Geometry check sheet. Reference: the model listing, model coordinates, mm. A direction names the side the tool comes from. Round coordinates to 2 decimals unless told otherwise and drop trailing zeros. Write each loop counter-clockwise with the first axis right and the second up, starting at its lowest first coordinate (ties: lowest second). Pieces come first, ordered by that corner, then holes. Notation, with made-up numbers: (-9.75, -14) - (42.25, -14) arc R4 cw to (42.25, -8) - close; hole circle Ø7 at (-14.5, 30). An arc over 180 degrees is marked (long way). Return JSON: item names as keys, results as strings.
```python
from build123d import *

# Parameters (mm, degrees)
SKETCH1_W           = 75
SKETCH1_H           = 180
BOSS_EXTRUDE1_DEPTH = 6
FILLET1_R           = 10
SKETCH2_R           = 10.5
SKETCH2_R_2         = 1.25
SKETCH2_R_3         = 1.65
CUT_EXTRUDE1_DEPTH  = 10
CUT_EXTRUDE2_DEPTH  = 3
SKETCH5_R           = 3.5
SKETCH5_W           = 47
SKETCH5_H           = 60
CUT_EXTRUDE3_DEPTH  = 3
FILLET2_R           = 10
CHAMFER1_SIZE       = 3
SKETCH6_W           = 5
SKETCH6_H           = 10
BOSS_EXTRUDE2_DEPTH = 6
CHAMFER2_SIZE       = 6


with BuildPart() as part:
    # Sketch1 → Boss-Extrude1 (new body)
    with BuildSketch(Plane(origin=(0, 0, 0), x_dir=(1, 0, 0), z_dir=(0, 1, 0))):
        Rectangle(SKETCH1_W, SKETCH1_H)
    extrude(amount=BOSS_EXTRUDE1_DEPTH)

    # Fillet1
    fillet1_edges = [part.edges().sort_by_distance(p)[0] for p in [
        (-37.5, 3, -90),
        (37.5, 3, -90),
        (37.5, 3, 90),
        (-37.5, 3, 90),
    ]]
    fillet(fillet1_edges, radius=FILLET1_R)

    # Sketch2 → Cut-Extrude1 (cut)
    with BuildSketch(Plane(origin=(0, 6, 0), x_dir=(1, 0, 0), z_dir=(0, 1, 0))):
        with Locations(Location((0, 0, 0), (0, 0, 270))):
            Circle(SKETCH2_R)
        with Locations(Location((-11, 8, 0), (0, 0, 270))):
            Circle(SKETCH2_R_2)
        with Locations(Location((11, 8, 0), (0, 0, 270))):
            Circle(SKETCH2_R_2)
        with Locations(Location((-11, -32, 0), (0, 0, 270))):
            Circle(SKETCH2_R_2)
        with Locations(Location((11, -32, 0), (0, 0, 270))):
            Circle(SKETCH2_R_2)
        with Locations(Location((-28, -70, 0), (0, 0, 270))):
            Circle(SKETCH2_R_3)
        with Locations(Location((28, -70, 0), (0, 0, 270))):
            Circle(SKETCH2_R_3)
        with Locations(Location((-28, 70, 0), (0, 0, 270))):
            Circle(SKETCH2_R_3)
        with Locations(Location((28, 70, 0), (0, 0, 270))):
            Circle(SKETCH2_R_3)
        with Locations(Location((-28, 10, 0), (0, 0, 270))):
            Circle(SKETCH2_R_3)
        with Locations(Location((-28, -10, 0), (0, 0, 270))):
            Circle(SKETCH2_R_3)
        with Locations(Location((28, 10, 0), (0, 0, 270))):
            Circle(SKETCH2_R_3)
        with Locations(Location((28, -10, 0), (0, 0, 270))):
            Circle(SKETCH2_R_3)
        with Locations(Location((-28, 30, 0), (0, 0, 270))):
            Circle(SKETCH2_R_3)
        with Locations(Location((28, 30, 0), (0, 0, 270))):
            Circle(SKETCH2_R_3)
        with Locations(Location((28, -30, 0), (0, 0, 270))):
            Circle(SKETCH2_R_3)
        with Locations(Location((-28, -30, 0), (0, 0, 270))):
            Circle(SKETCH2_R_3)
    extrude(amount=-CUT_EXTRUDE1_DEPTH, mode=Mode.SUBTRACT)

    # Sketch4 → Cut-Extrude2 (cut)
    with BuildSketch(Plane.XZ):
        Polygon((-28, 6.766838493), (-25.2, 8.383419246), (-25.2, 11.616580754), (-28, 13.233161507), (-30.8, 11.616580754), (-30.8, 8.383419246), align=None)
        Polygon((-27.920583163, -13.232185994), (-25.161136401, -11.547315999), (-25.240553238, -8.315130005), (-28.079416837, -6.767814006), (-30.838863599, -8.452684001), (-30.759446762, -11.684869995), align=None)
        Polygon((28, -13.233161507), (30.8, -11.616580754), (30.8, -8.383419246), (28, -6.766838493), (25.2, -8.383419246), (25.2, -11.616580754), align=None)
        Polygon((28, 6.766838493), (30.8, 8.383419246), (30.8, 11.616580754), (28, 13.233161507), (25.2, 11.616580754), (25.2, 8.383419246), align=None)
        Polygon((28, 66.766838493), (30.8, 68.383419246), (30.8, 71.616580754), (28, 73.233161507), (25.2, 71.616580754), (25.2, 68.383419246), align=None)
        Polygon((-28, 66.766838493), (-25.2, 68.383419246), (-25.2, 71.616580754), (-28, 73.233161507), (-30.8, 71.616580754), (-30.8, 68.383419246), align=None)
        Polygon((28, -73.233161507), (30.8, -71.616580754), (30.8, -68.383419246), (28, -66.766838493), (25.2, -68.383419246), (25.2, -71.616580754), align=None)
        Polygon((-28, -73.233161507), (-25.2, -71.616580754), (-25.2, -68.383419246), (-28, -66.766838493), (-30.8, -68.383419246), (-30.8, -71.616580754), align=None)
    extrude(amount=-CUT_EXTRUDE2_DEPTH, mode=Mode.SUBTRACT)

    # Sketch5 → Cut-Extrude3 (cut)
    with BuildSketch(Plane(origin=(0, 6, 0), x_dir=(1, 0, 0), z_dir=(0, 1, 0))):
        with Locations((-11, 8)):
            Circle(SKETCH5_R)
        with Locations((11, 8)):
            Circle(SKETCH5_R)
        with Locations((0, 50)):
            Rectangle(SKETCH5_W, SKETCH5_H)
        with Locations((0, -50)):
            Rectangle(SKETCH5_W, SKETCH5_H)
    extrude(amount=-CUT_EXTRUDE3_DEPTH, mode=Mode.SUBTRACT)

    # Fillet2
    fillet2_edges = [part.edges().sort_by_distance(p)[0] for p in [
        (-7.57722899, 4.5, -7.268810139),
        (-9.249798037, 4.5, -4.969027699),
        (9.249798037, 4.5, -4.969027699),
        (7.57722899, 4.5, -7.268810139),
    ]]
    fillet(fillet2_edges, radius=FILLET2_R)

    # Chamfer1
    chamfer1_edges = [part.edges().sort_by_distance(p)[0] for p in [
        (0, 3, 80),
        (0, 3, -80),
        (0, 3, -20),
        (0, 3, 20),
    ]]
    chamfer(chamfer1_edges, length=CHAMFER1_SIZE - 0.0001)  # a hair under: the kernel refuses the full size

    # Sketch6 → Boss-Extrude2 (add)
    with BuildSketch(Plane(origin=(0, 6, 0), x_dir=(1, 0, 0), z_dir=(0, 1, 0))):
        with Locations((-21, 85)):
            Rectangle(SKETCH6_W, SKETCH6_H)
        with Locations((21, -85)):
            Rectangle(SKETCH6_W, SKETCH6_H)
        with Locations((21, 85)):
            Rectangle(SKETCH6_W, SKETCH6_H)
        with Locations((-21, -85)):
            Rectangle(SKETCH6_W, SKETCH6_H)
    extrude(amount=BOSS_EXTRUDE2_DEPTH)

    # Chamfer2
    chamfer2_edges = [part.edges().sort_by_distance(p)[0] for p in [
        (21, 12, 90),
        (-21, 12, -90),
        (21, 12, -90),
        (-21, 12, 90),
    ]]
    chamfer(chamfer2_edges, length=CHAMFER2_SIZE)


solid = part.part
```
(1) Section check C-C, the plane z = 70. Enter the section's corners in (x, y), plus the area to 3 significant figures.
Response values:
{"outline": "(-37.5, 0) - (-30.8, 0) - (-30.8, 3) - (-29.65, 3) - (-29.65, 6) - (-37.5, 6) - close; (-26.35, 3) - (-25.2, 3) - (-25.2, 0) - (25.2, 0) - (25.2, 3) - (26.35, 3) - (26.35, 6) - (23.5, 6) - (23.5, 3) - (-23.5, 3) - (-23.5, 6) - (-26.35, 6) - close; (29.65, 3) - (30.8, 3) - (30.8, 0) - (37.5, 0) - (37.5, 6) - (29.65, 6) - close", "area": "256 mm^2"}
(2) Release check for a two-part mould opening along X. For faces 5 (the face through (-25.2, 1, -70)), 6 (the face through (21, 9, 87)), 7 (the face through (37.5, 3, 1)), 8 (the face through (29.636, 3.042, -30.215)) record: pulls with the +X half, pulls with the -X half, needs draft (parallel to the pull), parting line crosses it, or undercut.
Response values:
{"face 5": "undercut", "face 6": "needs draft", "face 7": "pulls with the +X half", "face 8": "undercut"}
(3) Material ranges on line 1 along X through (y, z) = (1.2, 30); line 2 along Z through (x, y) = (-7, 5.25); line 3 along Z through (x, y) = (7, 5.5), recorded low to high. Write a range as [from, to].
Response values:
{"line 1": "x = [-37.5, -29.65], [-26.35, 26.35], [29.65, 37.5]", "line 2": "z = [-90, -79.25], [-20.75, -10.21], [7.83, 20.75], [79.25, 90]", "line 3": "z = [-90, -79.5], [-20.5, -10.21], [7.83, 20.5], [79.5, 90]"}
(4) Gauge pin test, flat ends, axial feed: pin 1 (14 mm diameter, centred on x = -7, z = 47.5, fed in from +Y); pin 2 (5 mm diameter, centred on y = 8, z = -84, fed in from -X); pin 3 (6 mm diameter, centred on x = 15, y = 8, fed in from -Z); pin 4 (8 mm diameter, centred on x = -27, z = 30, fed in from +Y). Record the tip position at first contact, or that the pin passes through.
Response values:
{"pin 1": "stops at y = 3", "pin 2": "stops at x = -37.18", "pin 3": "stops at z = -90", "pin 4": "stops at y = 6"}
(5) Section check A-A, the plane y = 10. Enter the section's corners in (x, z), plus the area to 3 significant figures.
Response values:
{"outline": "(-23.5, -86) - (-18.5, -86) - (-18.5, -80) - (-23.5, -80) - close; (-23.5, 80) - (-18.5, 80) - (-18.5, 86) - (-23.5, 86) - close; (18.5, -86) - (23.5, -86) - (23.5, -80) - (18.5, -80) - close; (18.5, 80) - (23.5, 80) - (23.5, 86) - (18.5, 86) - close", "area": "120 mm^2"}
(6) Access from +Z, -Z, +X, -X, +Y, -Y to the whole of each face (thin tool, end or side, straight path). Record for faces 1 (the face through (19, 9, -80)), 2 (the face through (0, 6, 85)), 3 (the face through (25.2, 1, -10)), 4 (the face through (0, 3, 50)).
Response values:
{"face 1": "+X, -X, +Y", "face 2": "+Z, -Z, +Y", "face 3": "-Y", "face 4": "+Y"}
